Build history of the part. All positions in model axes, mm. A direction names the side the tool comes from. Round coordinates to 2 decimals unless told otherwise and drop trailing zeros. Write each question's results on one line, items separated by ' | '. Start each with the question number.
Autodesk Fusion 360 part; units mm, degrees
sketch "Skizze1" plane through (0, 0, 0) normal (0, 0, 1) x (1, 0, 0)
  line L0 (0, 0) -> (60, 0)
  line L1 (60, 0) -> (60, 110)
  line L2 (60, 110) -> (0, 110)
  line L3 (0, 110) -> (0, 0)
  circle A0 centre (10, 105) radius 2
  circle A1 centre (53, 105) radius 2
  circle A2 centre (10, 5) radius 2
  circle A3 centre (53, 5) radius 2
  line L4 (5, 95) -> (55, 95)
  line L5 (55, 95) -> (55, 15)
  line L6 (55, 15) -> (5, 15)
  line L7 (5, 15) -> (5, 95)
  dimension "d1" = 60
  dimension "d2" = 110
  dimension "d3" = 43
  dimension "d4" = 100
  dimension "d5" = 4
  dimension "d6" = 4
  dimension "d7" = 4
  dimension "d8" = 4
  dimension "d9" = 50
  dimension "d10" = 80
ref_plane "Arbeitsebene1" through (30, 55, 40) normal (0, 0, 1) x (1, 0, 0)
sketch "Skizze2" plane through (0, 0, 40) normal (0, 0, 1) x (1, 0, 0)
  line L0 (5, 95) -> (85, 95)
  line L1 (85, 95) -> (85, 15)
  line L2 (85, 15) -> (5, 15)
  line L3 (5, 15) -> (5, 95)
  circle A0 centre (81, 19) radius 2
  circle A1 centre (9, 19) radius 2
  circle A2 centre (9, 91) radius 2
  circle A3 centre (81, 91) radius 2
  circle A4 centre (45, 55) radius 39
  dimension "d12" = 80
  dimension "d13" = 80
  dimension "d14" = 72
  dimension "d15" = 72
  dimension "d18" = 4
  dimension "d19" = 4
  dimension "d20" = 4
  dimension "d21" = 4
  dimension "d22" = 78
extrude "Extrusion1" add sketch "Skizze2" along normal blind 1 makes body 1
extrude "Extrusion2" add sketch "Skizze1" along normal blind 1 separate body makes body 2
sketch "Skizze3" plane through (0, 0, 1) normal (0, 0, 1) x (-1, 0, 0)
  circle A0 centre (-53, -5) radius 2
  circle A1 centre (-10, -105) radius 2
  line L0 (-55, -15) -> (-5, -15)
  line L1 (-5, -15) -> (-5, -95)
  line L2 (-5, -95) -> (-55, -95)
  line L3 (-55, -95) -> (-55, -15)
  circle A2 centre (-10, -5) radius 2
  circle A3 centre (-53, -105) radius 2
  line L4 (0, -110) -> (0, 0)
  line L5 (0, 0) -> (-60, 0)
  line L6 (-60, 0) -> (-60, -110)
  line L7 (-60, -110) -> (0, -110)
  line L8 (-5, -95) -> (-55, -95)
  line L9 (-55, -95) -> (-55, -15)
  line L10 (-55, -15) -> (-5, -15)
  line L11 (-5, -15) -> (-5, -95)
sketch "Skizze4" plane through (0, 0, 40) normal (0, 0, -1) x (1, 0, 0)
  circle A0 centre (9, -91) radius 2
  circle A1 centre (9, -19) radius 2
  circle A2 centre (45, -55) radius 39
  circle A3 centre (81, -91) radius 2
  circle A4 centre (81, -19) radius 2
  line L0 (85, -15) -> (5, -15)
  line L1 (5, -15) -> (5, -95)
  line L2 (5, -95) -> (85, -95)
  line L3 (85, -95) -> (85, -15)
  circle A5 centre (45, -55) radius 39
loft "Erhebung1" add profiles "Skizze3", "Skizze4" section 1 section 2 bodies 1 2
loft "Erhebung2" cut section 1 face at (50.4593, 44.7073, 40) section 2 face at (38.3333, 68.3333, 1) on bodies 1 bodies 1
extrude "Extrusion3" cut 4 faces at (9.0794, 18.5317, 40) (9.5113, 91.1239, 40) (80.8813, 90.5466, 40) (80.1558, 20.1279, 40) along direction (0, 0, -1) blind 3 on bodies 1 bodies 1
extrude "Extrusion4" cut 4 faces at (52.3408, 5.0994, 1) (53.6332, 104.277, 1) (10.637, 103.8966, 1) (10.4521, 6.4238, 1) along direction (0, 0, 1) blind 6 on bodies 1 bodies 1
1. 3-axis set-ups, long thin cutter, end or side, ignore diameter. For faces 3 (the face through (10, 103, 3)), 4 (the face through (9, 89, 39)), 5 (the face through (6, 49, 41)): which of +Z, -Z, +X, -X, +Y, -Y reach the whole face in a straight line?
2. Wall check: line 1 (Y direction, x = 10, z = 5); line 2 (Y direction, x = 53, z = 2); line 3 (X direction, y = 90.5, z = 22). Give the ranges that are in metal, low to high. Write a range as from..to.
3. Mould opens along Y. For faces 1 (the face through (10, 105, 7)), 2 (the face through (56, 56, 0)) say: pulls with the +Y half, pulls with the -Y half, needs draft (parallel to the pull), parting line crosses it, or undercut.
4. Flat gauge pins, fed straight in: pin 1 Ø6 at (x, z) = (56, 27.5) entering from +Y; pin 2 Ø0.8 at (x, z) = (35, 40.5) entering from +Y; pin 3 Ø1 at (x, y) = (65, 27.5) entering from +Z; pin 4 Ø4.5 at (x, y) = (53, 5.5) entering from -Z. Where does each tip first touch, or does it go through?
A:
1) face 3: -Z | face 4: +Z | face 5: +Z, +X, -X, +Y, -Y
2) line 1: y = 1.54..3, 7..15.57, 94.43..103, 107..108.46 | line 2: y = 0.38..3, 7..15.15, 94.85..103, 107..109.62 | line 3: x = 2.69..14.95, 61.2..73.46
3) face 1: undercut | face 2: needs draft
4) pin 1: stops at y = 100.96 | pin 2: stops at y = 95 | pin 3: stops at z = 22.79 | pin 4: stops at z = 0
